Could you check a few things on this model? Use its own coordinates, in mm. Face numbers are marked on the shaded views. Round coordinates to 2 decimals unless told otherwise and drop trailing zeros. Loops run counter-clockwise (first coordinate to the right, second up) from the corner with the lowest first, then second, coordinate; pieces in that order, holes last.
Autodesk Inventor part; units mm, degrees
ref_plane "YZ Plane" through (0, 0, 0) normal (1, 0, 0) x (0, 1, 0)
ref_plane "XZ Plane" through (0, 0, 0) normal (0, 1, 0) x (-1, 0, 0)
ref_plane "XY Plane" through (0, 0, 0) normal (0, 0, 1) x (1, 0, 0)
sketch "Sketch1" plane through (0, 0, 0) normal (0, 0, 1) x (1, 0, 0)
  circle A0 centre (0, 0) radius 5
  dimension "d0" = 10
extrude "Extrusion1" add sketch "Sketch1" along normal blind 2
sketch "Sketch2" plane through (0, 0, 2) normal (0, 0, 1) x (1, 0, 0)
  circle A0 centre (0, 0) radius 4
  dimension "d3" = 8
extrude "Extrusion2" add sketch "Sketch2" along normal blind 3
sketch "Sketch3" plane through (0, 0, 5) normal (0, 0, 1) x (1, 0, 0)
  circle A0 centre (0, 0) radius 5
extrude "Extrusion3" add sketch "Sketch3" along normal blind 2
fillet "Fillet1" radius 2 2 edges at (-4, 0, 2) (-4, 0, 5)
sketch "Sketch4" plane through (0, 0, 7) normal (0, 0, 1) x (1, 0, 0)
  circle A0 centre (0, 0) radius 1.25
  dimension "d9" = 2.5
extrude "Extrusion4" cut sketch "Sketch4" against normal blind 20
properties part number "pully"
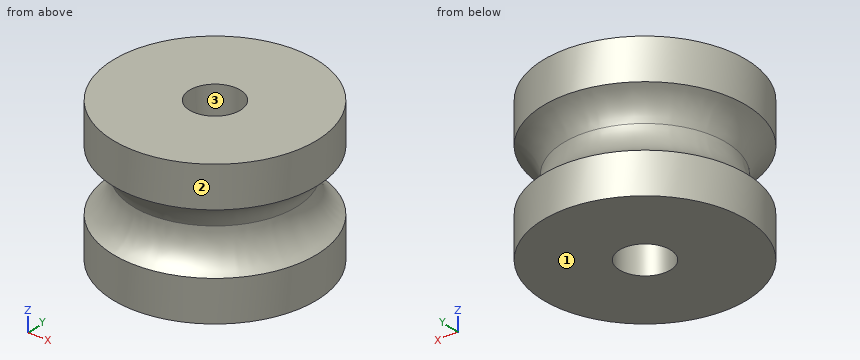
Item 1: If I drill on line 1 along Y through (x, z) = (0, 5.75); line 2 along Y through (x, z) = (0, 4.5); line 3 along X through (y, z) = (-0.5, 4), over which ranges is the centre line in solid material (lowest first)?
Results list:
line 1: y = -5 to -1.25, 1.25 to 5
line 2: y = -4.39 to -1.25, 1.25 to 4.39
line 3: x = -4.06 to -1.15, 1.15 to 4.06
Item 2: If we section it at C-C, the plane z = 5.5: Please give me the cut outline in (x, y).
Results list:
outline: circle Ø10 at (0, 0); hole circle Ø2.5 at (0, 0)
Item 3: If we section it at D-D, the plane z = 2.25: Please give me the cut outline in (x, y).
Results list:
outline: circle Ø9.31 at (0, 0); hole circle Ø2.5 at (0, 0)
Item 4: We'd pull the mould along X, two halves only. Please class the marked faces 1, 2 and 3: released by +X, released by -X, zero draft, split by the parting line, or undercut.
Results list:
face 1: zero draft
face 2: split by the parting line
face 3: undercut
Item 5: Will these pins go through, and if not, where does the flat tip stop? pin 1 (1.5 mm diameter, centred on x = -1, z = 3, fed in from +Y); pin 2 (4 mm diameter, centred on x = -1.5, z = 6, fed in from -Y).
Results list:
pin 1: stops at y = 4.56
pin 2: stops at y = -5
Item 6: If we section it at A-A, the plane y = 0: Please give me the cut outline in (x, z), then the cut area to 3 significant figures.
Results list:
outline: (-5, 0) - (-1.25, 0) - (-1.25, 7) - (-5, 7) - (-5, 5) arc R2 cw to (-4, 3.73) arc R2 cw to (-5, 2) - close; (1.25, 0) - (5, 0) - (5, 2) arc R2 cw to (4, 3.73) arc R2 cw to (5, 5) - (5, 7) - (1.25, 7) - close
area: 48.4 mm2
